Read the model definition and answer for the solid it produces. Units are mm, in the model's axes. Coordinates: 2 decimals unless noted, no trailing zeros. Write each loop counter-clockwise with the first axis right and the second up, starting at its lowest first coordinate (ties: lowest second). Pieces come first, ordered by that corner, then holes. Notation, with made-up numbers: (62, 10.5) - (89, 10.5) arc R22 ccw to (89, 41.5) - close; hole circle Ø2 at (79, 59). An arc over 180 degrees is marked (long way). Return JSON: item names as keys, results as strings.
```python
from build123d import *

# Parameters (mm, degrees)
BOSS_EXTRUDE1_DEPTH = 10


with BuildPart() as part:
    # Sketch1 → Boss-Extrude1 (new body)
    with BuildSketch(Plane(origin=(0, 0, 0), x_dir=(1, 0, 0), z_dir=(0, 1, 0))):
        Polygon((43.301270189, 75), (0, 0), (206.602540378, 0), (163.301270189, 75), align=None)
        Polygon((80.254006688, 60), (130.254006688, 60), (105.254006688, 16.698729811), align=None, mode=Mode.SUBTRACT)
        Polygon((125.601586083, 13.695227923), (150.601586083, 56.996498112), (175.601586083, 13.695227923), align=None, mode=Mode.SUBTRACT)
        Polygon((31.804368121, 15.086781489), (56.804368121, 58.388051678), (81.804368121, 15.086781489), align=None, mode=Mode.SUBTRACT)
    extrude(amount=BOSS_EXTRUDE1_DEPTH)


solid = part.part
```
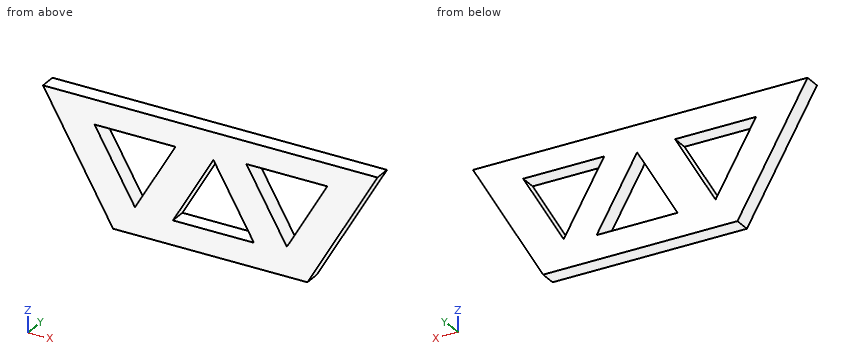
(1) Straight lines are drawn through the part: line 1 (X direction, y = 8.5, z = -42); line 2 (X direction, y = 1.75, z = -48.5); line 3 (Z direction, x = 126, y = 7). For each, find the intervals that lie inside material, in ascending order. Write a range as from..to.
Answer:
{"line 1": "24.25..47.34, 66.27..90.65, 119.86..141.94, 159.26..182.35", "line 2": "28..51.1, 62.51..86.89, 123.61..145.7, 155.51..178.6", "line 3": "-75..-60, -52.63..-14.39, -13.7..0"}
(2) A cutting plane is placed at D-D (x = 96). Determine the outline of the cut face in (y, z), and give its area (3 significant figures).
Answer:
{"outline": "(0, -75) - (10, -75) - (10, -60) - (0, -60) - close; (0, -32.73) - (10, -32.73) - (10, 0) - (0, 0) - close", "area": "477 mm²"}
(3) A cutting plane is placed at C-C (x = 65.5). Determine the outline of the cut face in (y, z), and give its area (3 significant figures).
Answer:
{"outline": "(0, -75) - (10, -75) - (10, -43.33) - (0, -43.33) - close; (0, -15.09) - (10, -15.09) - (10, 0) - (0, 0) - close", "area": "468 mm²"}
(4) A cutting plane is placed at B-B (y = 4.5). Determine the outline of the cut face in (x, z).
Answer:
{"outline": "(0, 0) - (43.3, -75) - (163.3, -75) - (206.6, 0) - close; hole (31.8, -15.09) - (56.8, -58.39) - (81.8, -15.09) - close; hole (80.25, -60) - (130.25, -60) - (105.25, -16.7) - close; hole (125.6, -13.7) - (150.6, -57) - (175.6, -13.7) - close"}
(5) A cutting plane is placed at A-A (z = -36). Determine the outline of the cut face in (x, y).
Answer:
{"outline": "(20.78, 0) - (43.88, 0) - (43.88, 10) - (20.78, 10) - close; (69.73, 0) - (94.11, 0) - (94.11, 10) - (69.73, 10) - close; (116.4, 0) - (138.48, 0) - (138.48, 10) - (116.4, 10) - close; (162.72, 0) - (185.82, 0) - (185.82, 10) - (162.72, 10) - close"}
(6) A flat-ended cylindrical pin translates along its axis: P1, Ø6, axis at x = 112.5, z = -34.5, coming from the -Y side. Find the tip coordinate at first contact, or state that the pin passes through.
Answer:
{"P1": "y = 0"}
